For this review, take the finished solid that the model builds, in its own axes (mm). Face numbers are marked on the shaded views. A direction names the side the tool comes from. Round coordinates to 2 decimals unless told otherwise and drop trailing zeros. Write each loop counter-clockwise with the first axis right and the second up, starting at its lowest first coordinate (ties: lowest second). Pieces come first, ordered by that corner, then holes.
from build123d import *

# Parameters (mm, degrees)
F0_W     = 203.2
F0_H     = 101.6
F1_DEPTH = 25.4
F3_DEPTH = 38.1
F4_R     = 33.39551
F5_DEPTH = 134.62


with BuildPart() as f1:
    # F0 (on Front) → F1 (new body)
    with BuildSketch(Plane.XZ):
        with Locations((-22.587857, 43.542857)):
            Rectangle(F0_W, F0_H)
    extrude(amount=F1_DEPTH)

    # F2 (on face) → F3 (join)
    with BuildSketch(Plane.XZ.offset(25.4)):
        Polygon((0, -7.257143), (-124.187857, 94.342857), (-124.187857, -7.257143), align=None)
    extrude(amount=F3_DEPTH)

    # F4 (on face) → F5 (cut)
    with BuildSketch(Plane.XZ.offset(63.5)):
        with Locations((-44.81934, 40.134594)):
            Circle(F4_R)
    extrude(amount=-F5_DEPTH, mode=Mode.SUBTRACT)


solid = f1.part
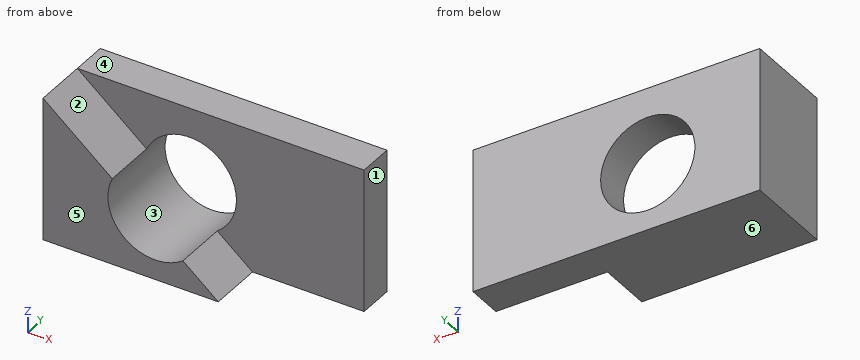
(1) For the marked faces 1 and 2, list the 3-axis set-ups (+Z, -Z, +X, -X, +Y, -Y) from which the entire face can be reached by the end or side of a thin tool; tool diameter is ignored.
Geometry check:
face 1: +Z, -Z, +X, +Y, -Y
face 2: +Z, +X, -Y
(2) We need section D-D, the plane z = 76. Give the boundary of the cut face in (x, y), and give its area (3 significant figures).
Geometry check:
outline: (-124.19, -63.5) - (-101.77, -63.5) - (-101.77, -25.4) - (79.01, -25.4) - (79.01, 0) - (-124.19, 0) - close
area: 6,020 mm2
(3) For line 1 along Y through (x, z) = (-79, 72); line 2 along Z through (x, y) = (-46, -12.5); line 3 along Z through (x, y) = (-60.5, -12), list the stretches that pass through material, from the lowest coordinate up.
Geometry check:
line 1: y = -25.4 to 0
line 2: z = -7.26 to 6.76, 73.51 to 94.34
line 3: z = -7.26 to 10.65, 69.62 to 94.34
(4) We need section C-C, the plane y = -5.5. Give the boundary of the cut face in (x, z).
Geometry check:
outline: (-124.19, -7.26) - (79.01, -7.26) - (79.01, 94.34) - (-124.19, 94.34) - close; hole circle Ø66.79 at (-44.82, 40.13)
(5) Mouldability with a two-part tool opening along Z and no side actions: class the marked faces 3, 4, 5 and 6 as pulls with the +Z half, pulls with the -Z half, needs draft (parallel to the pull), parting line crosses it, or undercut.
Geometry check:
face 3: undercut
face 4: pulls with the +Z half
face 5: needs draft
face 6: pulls with the -Z half
(6) We need section A-A, the plane z = 27.5. Give the boundary of the cut face in (x, y), and give its area (3 significant figures).
Geometry check:
outline: (-124.19, -63.5) - (-75.73, -63.5) - (-75.73, 0) - (-124.19, 0) - close; (-13.91, -25.4) - (79.01, -25.4) - (79.01, 0) - (-13.91, 0) - close
area: 5,440 mm2
(7) For pin 1 Ø8 at (x, z) = (-34, 81.5) entering from +Y; pin 2 Ø1 at (x, y) = (-78, -53) entering from +Z; pin 3 Ø1 at (x, z) = (-38, 81) entering from -Y; pin 4 Ø4 at (x, y) = (-100.5, -55) entering from +Z, all flat-tipped, find the tip position at first contact; note any pin that passes through.
Geometry check:
pin 1: stops at y = 0
pin 2: stops at z = 56.96
pin 3: stops at y = -25.4
pin 4: stops at z = 76.6
(8) We need section B-B, the plane x = -53.5. Give the boundary of the cut face in (y, z).
Geometry check:
outline: (-63.5, -7.26) - (0, -7.26) - (0, 7.89) - (-63.5, 7.89) - close; (-25.4, 72.38) - (0, 72.38) - (0, 94.34) - (-25.4, 94.34) - close
